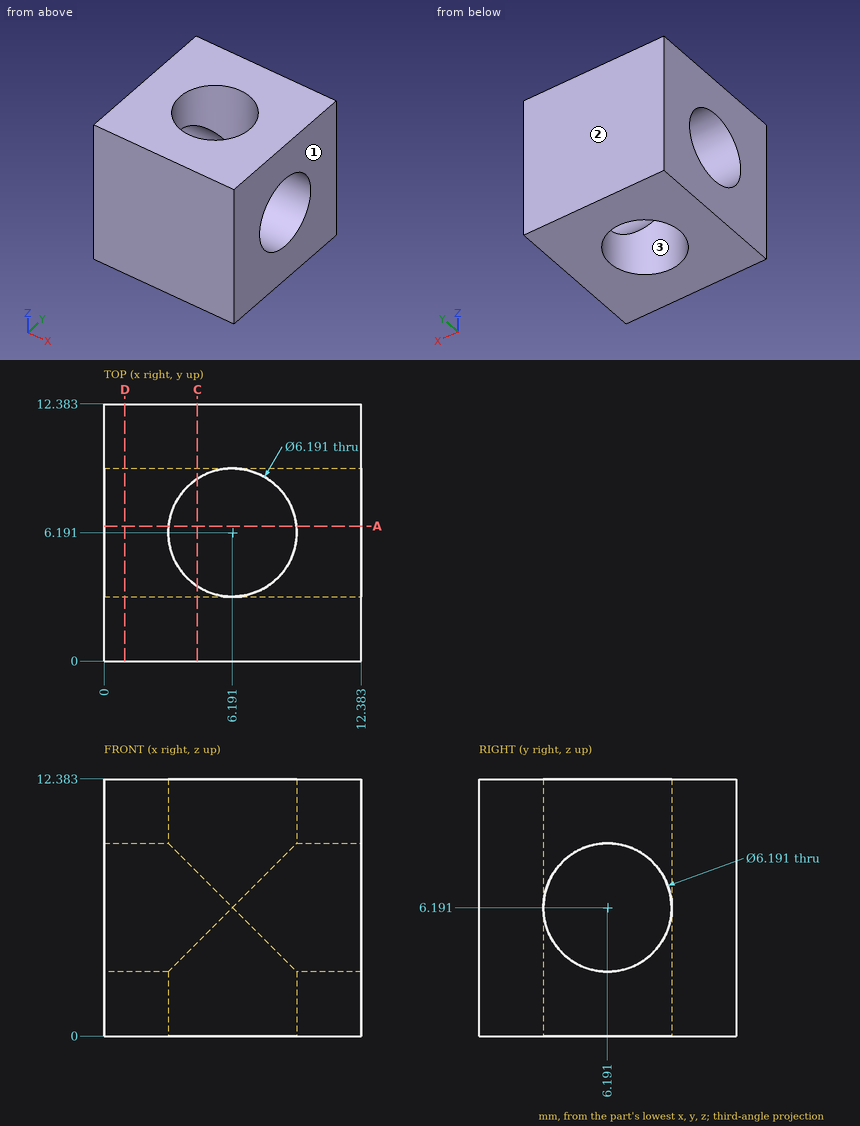
Drawing for the job (mm, zero at the part's lowest x, y, z). Coordinates: 2 decimals unless noted, no trailing zeros. Order: outer loops, then holes, each group sorted by start corner. A loop starts at its lowest first (then second) coordinate and runs counter-clockwise, first axis right, second up. Notation, with made-up numbers: (-5, 68) - (31, 68) arc R19 cw to (31, 95) - close; hole circle Ø10 at (43.25, 73). An arc over 180 degrees is marked (long way). Use a Markdown table: item, result. Add a question column.
(1) Drill centre lines: line 1 along Y through (x, z) = (1.25, 4.25) (1 decimal); line 2 along Y through (x, z) = (6.75, 11.75) (1 decimal); line 3 along Z through (x, y) = (2.5, 4.5) (1 decimal). Where is each one in solid material? Low to high. Write a range as [from, to].
(2) Saw through at C-C (x = 4.5). Give the cut face in (y, z) (1 decimal).
(3) Pull direction Y, two halves, no side cores. Call the marked faces 1, 2 and 3: +Y half, -Y half, draft (parallel to the pull), parting line (faces both ways), or undercut.
(4) Saw through at D-D (x = 1). Give the cut face in (y, z) (1 decimal).
(5) Saw through at A-A (y = 6.5). Give the cut face in (x, z).
Solved:
| question | item | result |
|---|---|---|
| 1 | line 1 | y = [0, 3.8], [8.6, 12.4] |
| 1 | line 2 | y = [0, 3.1], [9.2, 12.4] |
| 1 | line 3 | z = [0, 3.6], [8.8, 12.4] |
| 2 | outline | (0, 0) - (3.6, 0) - (3.6, 4.5) arc R3.1 cw to (3.6, 7.9) - (3.6, 12.4) - (0, 12.4) - close; (8.8, 0) - (12.4, 0) - (12.4, 12.4) - (8.8, 12.4) - (8.8, 7.9) arc R3.1 cw to (8.8, 4.5) - close |
| 3 | face 1 | draft |
| 3 | face 2 | +Y half |
| 3 | face 3 | undercut |
| 4 | outline | (0, 0) - (12.4, 0) - (12.4, 12.4) - (0, 12.4) - close; hole circle Ø6.2 at (6.2, 6.2) |
| 5 | outline | (0, 0) - (3.11, 0) - (3.11, 3.11) - (0, 3.11) - close; (0, 9.27) - (3.11, 9.27) - (3.11, 12.38) - (0, 12.38) - close; (9.27, 0) - (12.38, 0) - (12.38, 3.11) - (9.27, 3.11) - close; (9.27, 9.27) - (12.38, 9.27) - (12.38, 12.38) - (9.27, 12.38) - close |
